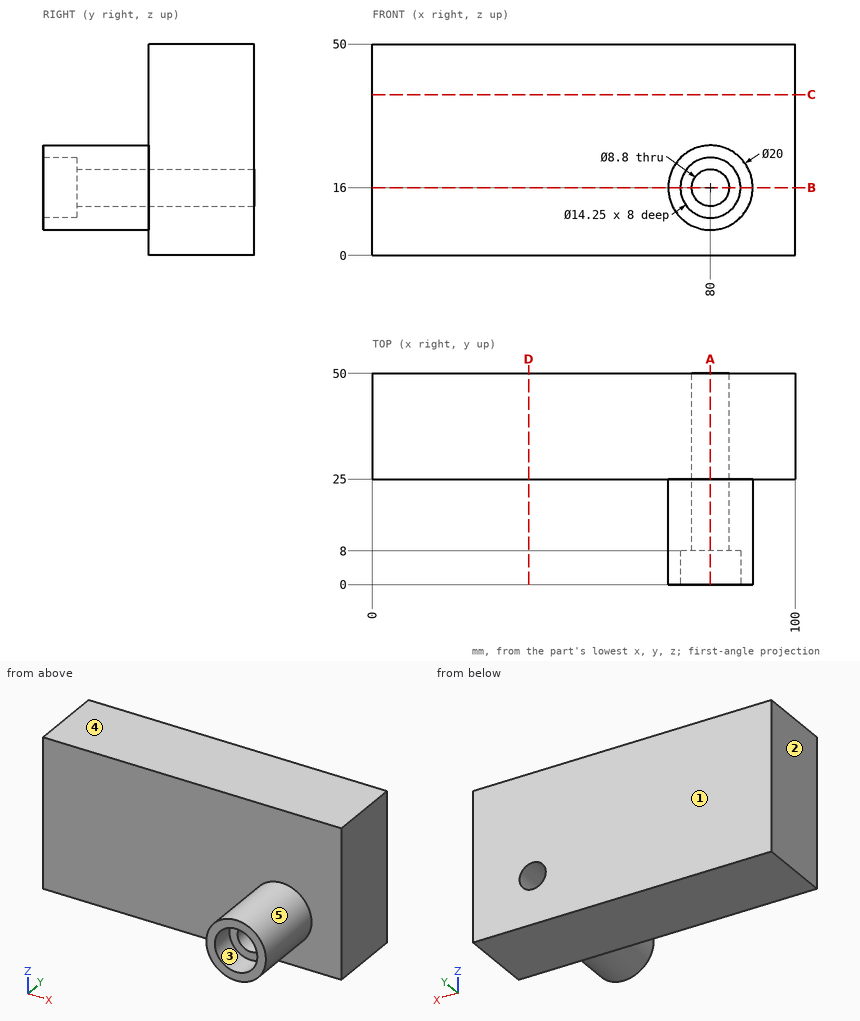
Geometry check sheet. Reference: drawing and pictorial views, mm from the part's lowest x, y, z. A direction names the side the tool comes from. Round coordinates to 2 decimals unless told otherwise and drop trailing zeros. Order: outer loops, then holes, each group sorted by start corner. A loop starts at its lowest first (then second) coordinate and runs counter-clockwise, first axis right, second up. Notation, with made-up numbers: (44, -36) -> (82, -36) arc R19 ccw to (82, -4) -> close; hole circle Ø7 at (35.5, 60). An arc over 180 degrees is marked (long way). One line per item, written item: value. Start each with the question number.
Q1. Mould release check, pull along X, two halves, no side actions. Record for the marked faces 1, 2 and 3: pulls with the +X half, pulls with the -X half, needs draft (parallel to the pull), parting line crosses it, or undercut.
Q2. Cross-section at A-A (x = 80). Record the boundary of the cut face in (y, z) (3 decimals).
Q3. Gauge pin test, flat ends, axial feed: pin 1 Ø10 at (y, z) = (11.5, 33) entering from -X (1 decimal); pin 2 Ø3 at (y, z) = (19.5, 16) entering from +X; pin 3 Ø11.5 at (x, z) = (80, 16) entering from -Y; pin 4 Ø5 at (y, z) = (14, 25.5) entering from -X. Record the tip position at first contact, or that the pin passes through.
Q4. Cross-section at C-C (z = 38). Record the boundary of the cut face in (x, y).
Q5. Set-up check for the marked faces 4 and 5: record each of +Z, -Z, +X, -X, +Y, -Y from which the full face is reachable in a straight line by a thin tool's end or side.
Q6. Cross-section at D-D (x = 37). Record the boundary of the cut face in (y, z).
Q7. Thickness scan on line 1 (Z direction, x = 80, y = 5) (3 decimals); line 2 (Z direction, x = 80, y = 39); line 3 (Y direction, x = 27.5, z = 33). Record the ranges inside material, lowest first.
Q8. Cross-section at B-B (z = 16). Record the boundary of the cut face in (x, y) (3 decimals), and give its area (3 significant figures).
Completed:
1. face 1: needs draft
1. face 2: pulls with the -X half
1. face 3: undercut
2. outline: (0, 6) -> (25, 6) -> (25, 0) -> (50, 0) -> (50, 11.6) -> (8, 11.6) -> (8, 8.875) -> (0, 8.875) -> close; (0, 23.125) -> (8, 23.125) -> (8, 20.4) -> (50, 20.4) -> (50, 50) -> (25, 50) -> (25, 26) -> (0, 26) -> close
3. pin 1: passes through
3. pin 2: stops at x = 90
3. pin 3: stops at y = 8
3. pin 4: stops at x = 72.86
4. outline: (0, 25) -> (100, 25) -> (100, 50) -> (0, 50) -> close
5. face 4: +Z, +X, -X, +Y, -Y
5. face 5: -Y
6. outline: (25, 0) -> (50, 0) -> (50, 50) -> (25, 50) -> close
7. line 1: z = 6 to 8.875, 23.125 to 26
7. line 2: z = 0 to 11.6, 20.4 to 50
7. line 3: y = 25 to 50
8. outline: (0, 25) -> (70, 25) -> (70, 0) -> (72.875, 0) -> (72.875, 8) -> (75.6, 8) -> (75.6, 50) -> (0, 50) -> close; (84.4, 8) -> (87.125, 8) -> (87.125, 0) -> (90, 0) -> (90, 25) -> (100, 25) -> (100, 50) -> (84.4, 50) -> close
8. area: 2,520 mm²
